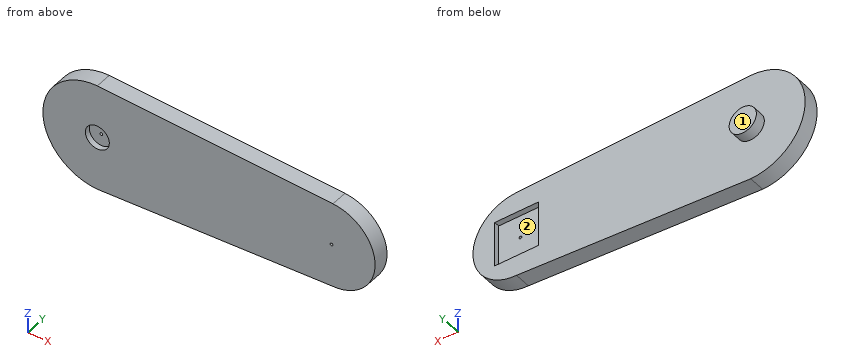
from build123d import *

# Parameters (mm, degrees)
CROQUIS1_R              = 1.25
SALIENTE_EXTRUIR1_DEPTH = 15
CROQUIS2_R              = 12.5
SALIENTE_EXTRUIR2_DEPTH = 10
CROQUIS3_R              = 11
CORTAR_EXTRUIR1_DEPTH   = 5
CROQUIS4_W              = 40
CROQUIS4_H              = 42
CORTAR_EXTRUIR2_DEPTH   = 5


with BuildPart() as part:
    # Croquis1 → Saliente-Extruir1 (new body)
    with BuildSketch(Plane(origin=(0, 0, 0), x_dir=(1, 0, 0), z_dir=(0, 1, 0))):
        with BuildLine():
            Line((0, 50), (215, 37.002241847))
            ThreePointArc((215, 37.002241847), (254.994732146, -2.34860444), (216.298136444, -42.976688126))
            Line((216.298136444, -42.976688126), (0, -50))
            ThreePointArc((0, -50), (-50, 0), (0, 50))
        make_face()
        with Locations(Location((0, 0, 0), (0, 0, 270))):
            Circle(CROQUIS1_R, mode=Mode.SUBTRACT)
        with Locations(Location((215, -2.997758153, 0), (0, 0, 270))):
            Circle(CROQUIS1_R, mode=Mode.SUBTRACT)
    extrude(amount=SALIENTE_EXTRUIR1_DEPTH)

    # Croquis2 → Saliente-Extruir2 (add)
    with BuildSketch(Plane(origin=(0, 15, 0), x_dir=(1, 0, 0), z_dir=(0, 1, 0))):
        with Locations(Location((0, 0, 0), (0, 0, 270))):
            Circle(CROQUIS2_R)
    extrude(amount=SALIENTE_EXTRUIR2_DEPTH)

    # Croquis3 → Cortar-Extruir1 (cut)
    with BuildSketch(Plane(origin=(0, 0, 0), x_dir=(-1, 0, 0), z_dir=(0, -1, 0))):
        with Locations(Location((0, 0, 0), (0, 0, 90))):
            Circle(CROQUIS3_R)
    extrude(amount=-CORTAR_EXTRUIR1_DEPTH, mode=Mode.SUBTRACT)

    # Croquis4 → Cortar-Extruir2 (cut)
    with BuildSketch(Plane(origin=(0, 15, 0), x_dir=(1, 0, 0), z_dir=(0, 1, 0))):
        with Locations((215, -2.997758153)):
            Rectangle(CROQUIS4_W, CROQUIS4_H)
    extrude(amount=-CORTAR_EXTRUIR2_DEPTH, mode=Mode.SUBTRACT)


solid = part.part
Here's how the part is built. I have some questions about the finished solid (model axes, mm). Face numbers are marked on the shaded views. Give positions to 0.01 mm unless a question says otherwise; leave off trailing zeros. Order: outer loops, then holes, each group sorted by start corner. A loop starts at its lowest first (then second) coordinate and runs counter-clockwise, first axis right, second up. Notation, with made-up numbers: M 12.5,-2 L 45.5,-2 A6 ccw 45.5,6 Z; hole C 42,11.25 d3. An arc over 180 degrees is marked long. Answer as a JSON object with one key per item and string values. Group by question number.
1) I'm going to push flat-ended pins straight in: pin 1 Ø2 at (y, z) = (5, -25.5) entering from -X; pin 2 Ø2.5 at (y, z) = (13.5, 6) entering from -X; pin 3 Ø1.5 at (x, z) = (215, 3) entering from -Y; pin 4 Ø2.5 at (x, y) = (220, 11.5) entering from -Z. Where does each tip first touch, or does it pass through?
2) Suppose I cut it at A-A, the plane x = 224.5. Write out the boundary of the cut face in (y, z), plus the area to 3 significant figures.
3) Suppose I cut it at B-B, the plane y = 22. Write out the boundary of the cut face in (x, z).
4) Suppose I cut it at D-D, the plane x = 83. Write out the boundary of the cut face in (y, z).
5) Suppose I cut it at C-C, the plane z = 32.5. Write out the boundary of the cut face in (x, y), plus the area to 3 significant figures.
6) Please list where these lines run through material, in increasing order: L1, parallel to Z at x = 0, y = 12.75; L2, parallel to Y at x = 171.5, z = 15; L3, parallel to Z at x = 215, y = 4.5. Write a range as [from, to].
7) We'd pull the mould along Z, two halves only. Please class the marked faces 1 and 2: pulls with the +Z half, pulls with the -Z half, needs draft (parallel to the pull), parting line crosses it, or undercut.
Results found:
{
 "1": {"pin 1": "x = -43.59", "pin 2": "x = -49.77", "pin 3": "through", "pin 4": "z = -36.83"},
 "2": {"outline": "M 0,-35.86 L 15,-35.86 L 15,-18 L 10,-18 L 10,24 L 15,24 L 15,41.85 L 0,41.85 Z", "area": "956 mm²"},
 "3": {"outline": "C 0,0 d25"},
 "4": {"outline": "M 0,-44.98 L 15,-44.98 L 15,47.3 L 0,47.3 Z"},
 "5": {"outline": "M -38,0 L 242.01,0 L 242.01,15 L -38,15 Z", "area": "4,200 mm²"},
 "6": {"L1": "[-50, -1.25], [1.25, 50]", "L2": "[0, 15]", "L3": "[-37, 1.75], [4.25, 43.02]"},
 "7": {"face 1": "needs draft", "face 2": "undercut"}
}
